Model file for the job. Use its own axes, mm. A direction names the side the tool comes from. Round coordinates to 2 decimals unless told otherwise and drop trailing zeros. Loops run counter-clockwise (first coordinate to the right, second up) from the corner with the lowest first, then second, coordinate; pieces in that order, holes last. Notation, with made-up numbers: (-13, 57.25) -> (40, 57.25) arc R7 cw to (40, 65.25) -> close; hole circle Ø3 at (84.5, -40). An arc over 180 degrees is marked (long way). Use a Markdown table: item, result.
from build123d import *

# Parameters (mm, degrees)
BOSS_EXTRUDE1_DEPTH = 3
SKETCH2_W           = 3
SKETCH2_H           = 6
SKETCH2_W_2         = 6
SKETCH2_H_2         = 3
BOSS_EXTRUDE2_DEPTH = 19
SKETCH3_W           = 78
SKETCH3_H           = 73
SKETCH3_W_2         = 72
SKETCH3_H_2         = 67
BOSS_EXTRUDE3_DEPTH = 3
SKETCH4_R           = 3.5
BOSS_EXTRUDE4_DEPTH = 3
CUT_EXTRUDE1_DEPTH  = 4
CUT_EXTRUDE2_DEPTH  = 3
SKETCH7_R           = 1.9
CUT_EXTRUDE3_DEPTH  = 3
SKETCH8_W           = 21
SKETCH8_H           = 27
SKETCH8_R           = 2
SKETCH8_R_2         = 4
BOSS_EXTRUDE5_DEPTH = 1.5
SKETCH9_R           = 1.5
SKETCH9_R_2         = 8.25
CUT_EXTRUDE4_DEPTH  = 3
SKETCH10_W          = 3
SKETCH10_H          = 6
CUT_EXTRUDE5_DEPTH  = 3
FILLET1_R           = 2.5


with BuildPart() as part:
    # Sketch1 → Boss-Extrude1 (new body)
    with BuildSketch(Plane(origin=(0, 0, 0), x_dir=(1, 0, 0), z_dir=(0, 1, 0))):
        Polygon((100, 24), (102, 24), (102, 0), (100, 0), (78, 0), (0, 0), (0, 15), (-26, 15), (-26, 58), (0, 58), (0, 73), (78, 73), (105, 73), (105, 46), (78, 46), (78, 24), align=None)
    extrude(amount=BOSS_EXTRUDE1_DEPTH)

    # Sketch2 → Boss-Extrude2 (add)
    with BuildSketch(Plane(origin=(0, 3, 0), x_dir=(1, 0, 0), z_dir=(0, 1, 0))):
        Polygon((0, 0), (3, 0), (6, 0), (6, 3), (3, 3), (3, 6), (0, 6), align=None)
        Polygon((78, 0), (75, 0), (72, 0), (72, 3), (75, 3), (75, 6), (78, 6), align=None)
        with Locations((1.5, 25.3333)):
            Rectangle(SKETCH2_W, SKETCH2_H)
        with Locations((1.5, 47.6663)):
            Rectangle(SKETCH2_W, SKETCH2_H)
        Polygon((0, 73), (3, 73), (6, 73), (36, 73), (39, 73), (39, 70), (36, 70), (17, 70), (3, 70), (3, 67), (0, 67), align=None)
        with Locations((27, 1.5)):
            Rectangle(SKETCH2_W_2, SKETCH2_H_2)
        with Locations((51, 1.5)):
            Rectangle(SKETCH2_W_2, SKETCH2_H_2)
        with Locations((76.5, 25.333)):
            Rectangle(SKETCH2_W, SKETCH2_H)
        Polygon((72, 73), (78, 73), (78, 70), (78, 67), (75, 67), (75, 70), (72, 70), align=None)
        with Locations((51, 71.5)):
            Rectangle(SKETCH2_W_2, SKETCH2_H_2)
    extrude(amount=BOSS_EXTRUDE2_DEPTH)

    # Sketch3 → Boss-Extrude3 (add)
    with BuildSketch(Plane(origin=(0, 22, 0), x_dir=(1, 0, 0), z_dir=(0, 1, 0))):
        with Locations((39, 36.5)):
            Rectangle(SKETCH3_W, SKETCH3_H)
        with Locations((39, 36.5)):
            Rectangle(SKETCH3_W_2, SKETCH3_H_2, mode=Mode.SUBTRACT)
    extrude(amount=BOSS_EXTRUDE3_DEPTH)

    # Sketch4 → Boss-Extrude4 (add)
    with BuildSketch(Plane(origin=(0, 3, 0), x_dir=(1, 0, 0), z_dir=(0, 1, 0))):
        with Locations((7.4, 65)):
            Circle(SKETCH4_R)
        Polygon((8.9, 65), (8.15, 66.299038106), (6.65, 66.299038106), (5.9, 65), (6.65, 63.700961894), (8.15, 63.700961894), align=None, mode=Mode.SUBTRACT)
        with Locations((7.4, 7.4)):
            Circle(SKETCH4_R)
        Polygon((8.9, 7.4), (8.15, 8.699038106), (6.65, 8.699038106), (5.9, 7.4), (6.65, 6.100961894), (8.15, 6.100961894), align=None, mode=Mode.SUBTRACT)
        with Locations((70.4, 7.4)):
            Circle(SKETCH4_R)
        Polygon((68.9, 7.4), (69.65, 6.100961894), (71.15, 6.100961894), (71.9, 7.4), (71.15, 8.699038106), (69.65, 8.699038106), align=None, mode=Mode.SUBTRACT)
        with Locations((60, 60)):
            Circle(SKETCH4_R)
    extrude(amount=BOSS_EXTRUDE4_DEPTH)

    # Sketch4_2 → Cut-Extrude1 (cut, through all)
    with BuildSketch(Plane(origin=(0, 3, 0), x_dir=(1, 0, 0), z_dir=(0, 1, 0))):
        Polygon((8.15, 63.700961894), (8.9, 65), (8.15, 66.299038106), (6.65, 66.299038106), (5.9, 65), (6.65, 63.700961894), align=None)
        Polygon((8.15, 6.100961894), (8.9, 7.4), (8.15, 8.699038106), (6.65, 8.699038106), (5.9, 7.4), (6.65, 6.100961894), align=None)
        Polygon((69.65, 8.699038106), (68.9, 7.4), (69.65, 6.100961894), (71.15, 6.100961894), (71.9, 7.4), (71.15, 8.699038106), align=None)
    extrude(amount=-CUT_EXTRUDE1_DEPTH, mode=Mode.SUBTRACT)

    # Sketch5 → Cut-Extrude2 (cut)
    with BuildSketch(Plane(origin=(0, 3, 0), x_dir=(1, 0, 0), z_dir=(0, 1, 0))):
        Polygon((80.601762475, 59.5), (79.351762475, 61.665063509), (76.851762475, 61.665063509), (75.601762475, 59.5), (76.851762475, 57.334936491), (79.351762475, 57.334936491), align=None)
    extrude(amount=-CUT_EXTRUDE2_DEPTH, mode=Mode.SUBTRACT)

    # Sketch7 → Cut-Extrude3 (cut)
    with BuildSketch(Plane(origin=(0, 0, -73), x_dir=(-1, 0, 0), z_dir=(0, 0, -1))):
        with Locations((-35.5, 20.1)):
            Circle(SKETCH7_R)
    extrude(amount=-CUT_EXTRUDE3_DEPTH, mode=Mode.SUBTRACT)

    # Sketch8 → Boss-Extrude5 (add)
    with BuildSketch(Plane(origin=(0, 25, 0), x_dir=(1, 0, 0), z_dir=(0, 1, 0))):
        with Locations((13.5, 56.5)):
            Rectangle(SKETCH8_W, SKETCH8_H)
        with Locations((14, 47)):
            Circle(SKETCH8_R, mode=Mode.SUBTRACT)
        with Locations((7.4, 65)):
            Circle(SKETCH8_R_2, mode=Mode.SUBTRACT)
    extrude(amount=-BOSS_EXTRUDE5_DEPTH)

    # Sketch9 → Cut-Extrude4 (cut)
    with BuildSketch(Plane(origin=(0, 3, 0), x_dir=(1, 0, 0), z_dir=(0, 1, 0))):
        with Locations((97, 20.5)):
            Circle(SKETCH9_R)
        with Locations((84, 3.5)):
            Circle(SKETCH9_R)
        with Locations((90.5, 12)):
            Circle(SKETCH9_R_2)
    extrude(amount=-CUT_EXTRUDE4_DEPTH, mode=Mode.SUBTRACT)

    # Sketch10 → Cut-Extrude5 (cut)
    with BuildSketch(Plane(origin=(0, 3, 0), x_dir=(1, 0, 0), z_dir=(0, 1, 0))):
        with Locations((64, 14.4)):
            Rectangle(SKETCH10_W, SKETCH10_H)
        with Locations((64, 50.4)):
            Rectangle(SKETCH10_W, SKETCH10_H)
        with Locations((14, 14.584176744)):
            Rectangle(SKETCH10_W, SKETCH10_H)
        with Locations((14, 50.584176744)):
            Rectangle(SKETCH10_W, SKETCH10_H)
    extrude(amount=-CUT_EXTRUDE5_DEPTH, mode=Mode.SUBTRACT)

    # Fillet1
    fillet1_edges = [part.edges().sort_by_distance(p)[0] for p in [
        (62.5, 3, -14.4),
        (15.5, 3, -50.584176744),
        (15.5, 3, -14.584176744),
        (62.5, 3, -50.4),
    ]]
    fillet(fillet1_edges, radius=FILLET1_R)


solid = part.part
Q1. Tool access for faces 3 (the face through (12.5, 2, -51)), 4 (the face through (54, 12, -71)), 5 (the face through (92, 1, -46)): list every direction of +Z, -Z, +X, -X, +Y, -Y with a clear straight run to the whole face (end or side of a thin tool).
Results list:
| item | result |
|---|---|
| face 3 | -Y |
| face 4 | +Z, -Z |
| face 5 | +X, +Y, -Y |
Q2. Pull direction X, two halves, no side cores. Call faces 1 (the face through (62, 2, -50)), 2 (the face through (1, 22, -14)): released by +X, released by -X, zero draft, split by the parting line, or undercut.
Results list:
| item | result |
|---|---|
| face 1 | undercut |
| face 2 | zero draft |
Q3. Band-saw the part on C-C, the plane y = 4.25. Give the number of separate pieces and of enclosed holes in the cut face, plus the area to 3 significant figures.
Results list:
| item | result |
|---|---|
| separate pieces | 14 |
| enclosed holes | 3 |
| area | 451 mm² |
Q4. Band-saw the part on D-D, the plane x = 35.5. Give the cut face in (y, z), plus the area to 3 significant figures.
Results list:
| item | result |
|---|---|
| outline | (0, -73) -> (18.2, -73) -> (18.2, -70) -> (3, -70) -> (3, 0) -> (0, 0) -> close; (22, -73) -> (25, -73) -> (25, -70) -> (22, -70) -> close; (22, -3) -> (25, -3) -> (25, 0) -> (22, 0) -> close |
| area | 283 mm² |
Q5. Band-saw the part on B-B, the plane z = -41.5. Give the cut face in (x, y), plus the area to 3 significant figures.
Results list:
| item | result |
|---|---|
| outline | (-26, 0) -> (78, 0) -> (78, 3) -> (-26, 3) -> close; (0, 22) -> (3, 22) -> (3, 25) -> (0, 25) -> close; (75, 22) -> (78, 22) -> (78, 25) -> (75, 25) -> close |
| area | 330 mm² |
Q6. Drill centre lines: L1, parallel to Z at x = 75.5, y = 6; L2, parallel to Z at x = 14, y = 24; L3, parallel to Y at x = 11, z = -48. Where is each one in solid material? Low to high. Write a range as from..to.
Results list:
| item | result |
|---|---|
| L1 | z = -73..-67, -28.33..-22.33, -6..0 |
| L2 | z = -73..-49, -45..-43, -3..0 |
| L3 | y = 0..3, 23.5..25 |
Q7. Flat gauge pins, fed straight in: pin 1 (1.6 mm diameter, centred on y = 24, z = -59.5, fed in from +X); pin 2 (5 mm diameter, centred on x = 6, z = -37, fed in from +Y); pin 3 (1.5 mm diameter, centred on y = 2, z = -15.5, fed in from +X); pin 4 (13 mm diameter, centred on x = 90.5, z = -12, fed in from +Y). Where does each tip first touch, or does it go through?
Results list:
| item | result |
|---|---|
| pin 1 | stops at x = 78 |
| pin 2 | stops at y = 3 |
| pin 3 | stops at x = 102 |
| pin 4 | passes through |
Q8. Band-saw the part on A-A, the plane x = 90.5. Give the cut face in (y, z).
Results list:
| item | result |
|---|---|
| outline | (0, -73) -> (3, -73) -> (3, -46) -> (0, -46) -> close; (0, -24) -> (3, -24) -> (3, -20.25) -> (0, -20.25) -> close; (0, -3.75) -> (3, -3.75) -> (3, 0) -> (0, 0) -> close |
